Autodesk Inventor part; units mm, degrees
ref_plane "Work Plane1" through (1.525, 0, 0) normal (0, 0, 1) x (1, 0, 0)
ref_plane "YZ Plane" through (0, 0, 0) normal (1, 0, 0) x (0, 1, 0)
ref_plane "XZ Plane" through (0, 0, 0) normal (0, 1, 0) x (-1, 0, 0)
sketch "Boceto1" plane through (0, 0, 0) normal (0, 0, 1) x (1, 0, 0)
  line L0 (0, 3.015) -> (0, 2)
  line L1 (2.1, 2) -> (8, 2)
  line L2 (8, 2) -> (8, 0)
  line L3 (8, 0) -> (-0.4001, 0)
  line L4 (-2.0801, 0) -> (9.68, 0)
  line L5 (-0.4001, 0) -> (-0.4001, 3.015)
  line L6 (-0.4001, 3.015) -> (0, 3.015)
  line L7 (2.1, 2) -> (1.6705, 2)
  line L8 (1.6705, 2) -> (0, 2)
  line L9 (0, -0.603) -> (0, 3.618)
  dimension "d0" = 8
  dimension "d1" = 5.9
  dimension "d2" = 4
  dimension "d9" = 0.4001
  dimension "d10" = 6.03
  dimension "d13" = 0.4295
  dimension "d14" = 4
revolve "Cuerpo" add sketch "Boceto1" angle 360 about axis through (8, 0, 0) along (-1, 0, 0)
sketch "Boceto2" plane through (-0.4001, 0, 0) normal (-1, 0, 0) x (0, 0, 1)
  line L0 (0, 4.0415) -> (3.5, 2.0207)
  line L1 (3.5, 2.0207) -> (3.5, -2.0207)
  line L2 (3.5, -2.0207) -> (0, -4.0415)
  line L3 (0, -4.0415) -> (-3.5, -2.0207)
  line L4 (-3.5, -2.0207) -> (-3.5, 2.0207)
  line L5 (-3.5, 2.0207) -> (0, 4.0415)
  point P0 (0, 0)
  point P1 (0, 0)
  dimension "d11" = 7
extrude "Cabeza" add sketch "Boceto2" along normal blind 2.4
sketch "Boceto4" plane through (0, 0, 0) normal (0, 0, 1) x (1, 0, 0)
  line L0 (-2.8001, 3.5) -> (-2.8001, 4.0415)
  line L1 (-2.8001, 4.0415) -> (-2.4875, 4.0415)
  line L2 (-2.4875, 4.0415) -> (-2.8001, 3.5)
  line L3 (-3.2801, 0) -> (0.0799, 0)
  line L4 (-0.4001, 4.0415) -> (-2.8001, 4.0415)
  line L5 (-2.8001, 2.0207) -> (-2.8001, 4.0415)
  dimension "d5" = 30
  dimension "d19" = 7
revolve "Chaflán1" cut sketch "Boceto4" angle 360 about axis through (-10, 0, 0) along (1, 0, 0)
thread "Rosca"
chamfer "Chaflán2" distance 0.4294 distance2 0.4295 1 edges at (8, -2, 0) measured on face at (8, 0.1822, 0.4036)
ref_plane "Work Plane1" through (1.525, 0, 0) normal (0, 0, 1) x (1, 0, 0)
equation "\"d0\" = NLG"
equation "\"d1\" = GEL"
equation "\"d2\" = GD"
equation "\"d10\" = SD2"
equation "\"d14\" = BDM"
equation "\"d11\" = SW"
equation "\"d3\" = KOH - SD"
equation "\"d5\" = ANG1"
equation "\"d19\" = SW0"
equation "\"d15\" = GEL"
equation "\"d6\" = -0.5 * SPD + 0.5 * GD"
equation "\"NLG\" = 8"
equation "\"GD\" = NND"
equation "\"BDM\" = NND"
equation "\"KOH\" = 2.8"
equation "\"GEL\" = 5.9"
equation "\"SW\" = 7"
equation "\"SW0\" = SW"
equation "\"SPD\" = NND - 1.2269 * PTC"
equation "\"SD2\" = 6.03"
equation "\"SD\" = 0.4"
equation "\"ANG1\" = 30deg"
equation "\"GAL\" = 0.61345 * PTC"
equation "\"GUL\" = 0.61345 * PTC"
equation "\"RR\" = 0.2"
equation "\"GD1\" = THREADDIA - 1.2269 * PTC"
equation "\"THREADDIA\" = 4"
equation "\"SDH\" = SD2"
equation "\"SDHG\" = 2.1"
equation "\"TOA\" = 30deg"
equation "\"PTC\" = 0.7"
equation "\"NND\" = 4"
equation "\"E0\" = 8.085"
properties part number "ISO 4017 - M4 x 8" material "Acero inoxidable, 440C"
Source: CAD feature listing. Evaluate the final solid. Frame: model axes, mm. A direction names the side the tool comes from. Give positions to 0.01 mm unless a question says otherwise; leave off trailing zeros. Loops run counter-clockwise (first coordinate to the right, second up) from the corner with the lowest first, then second, coordinate; pieces in that order, holes last. Notation, with made-up numbers: (-31.75, 5) -> (-19.75, 5) arc R11 cw to (-19.75, 25) -> close; hole circle Ø3 at (-23.75, 63.25). An arc over 180 degrees is marked (long way). Put each result on its own line as item: value. Start each with the question number.
1) Contact query for flat-ended pins moving along their axis: P1, Ø1, axis at y = -1.5, z = 1.5, coming from the +X side; P2, Ø3, axis at x = 2, y = -1.5, coming from the +Z side; P3, Ø4, axis at x = 7, z = -0.5, coming from the -Y side. Output: stop coordinate, or through.
2) Cut plane B-B (x = 2). Return loops of the section in (y, z), then the cut area to 3 significant figures.
3) Material intervals for probe 1 along X at (y, z) = (-1.75, -2.75); probe 2 along Y at (x, z) = (-1.25, -1.75); probe 3 along X at (y, z) = (2.5, 0), sorted ascending.
4) Cut plane A-A (x = -1). Return loops of the section in (y, z).
5) Reachability of faces 1 (the face through (-2.724, 3.632, -0.009)), 2 (the face through (-0.4, -3, -1.1)) from +Z, -Z, +X, -X, +Y, -Y: full face, straight path, thin tool, end or side. Return the list, or none.
Results are:
1. P1: stops at x = 7.95
1. P2: stops at z = 2
1. P3: stops at y = -2
2. outline: circle Ø4 at (0, 0)
2. area: 12.6 mm2
3. probe 1: x = -2.8 to -0.4
3. probe 2: y = -3.03 to 3.03
3. probe 3: x = -2.8 to 0
4. outline: (-4.04, 0) -> (-2.02, -3.5) -> (2.02, -3.5) -> (4.04, 0) -> (2.02, 3.5) -> (-2.02, 3.5) -> close
5. face 1: -X, +Y
5. face 2: +X
